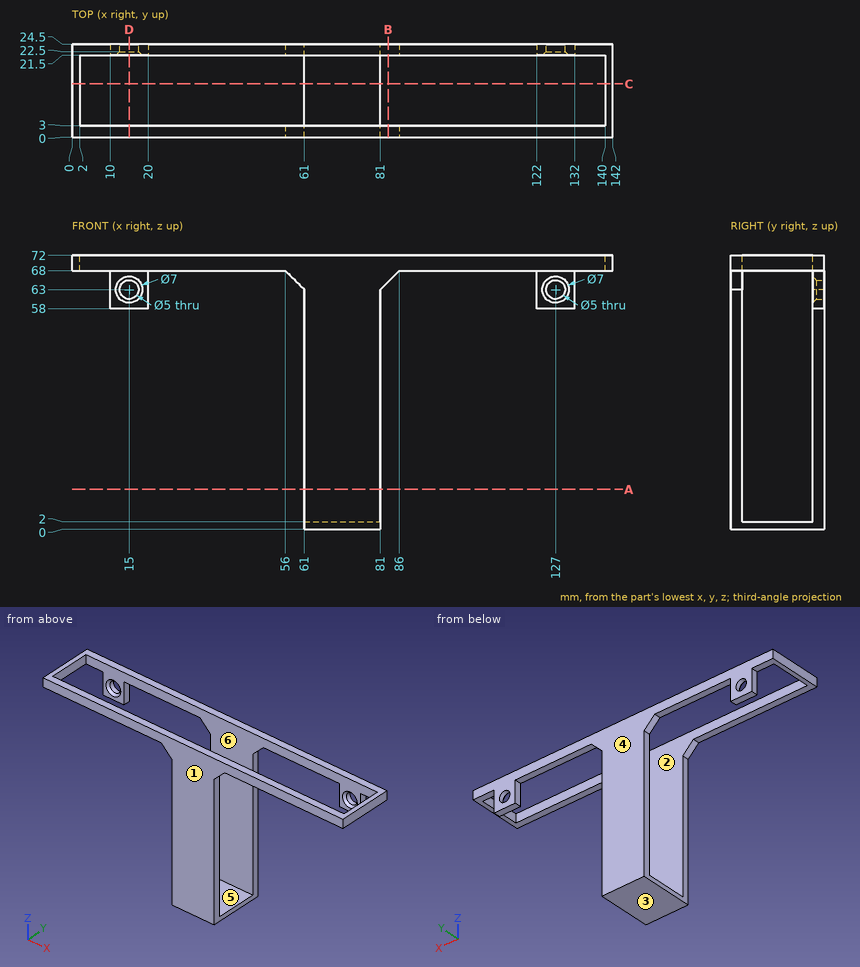
Geometry: see drawing. Coordinates: mm, zero at the bounding-box minimum. A direction names the side the tool comes from. Give positions to 0.01 mm unless a question says otherwise; leave off trailing zeros. Order: outer loops, then holes, each group sorted by start corner. A loop starts at its lowest first (then second) coordinate and runs counter-clockwise, first axis right, second up. Notation, with made-up numbers: (19.25, 84.25) -> (78.25, 84.25) arc R14 ccw to (78.25, 96.25) -> close; hole circle Ø6 at (-19, 52.5). An arc over 180 degrees is marked (long way). Write each question's results on one line, items separated by ' | '.
1) Cut plane D-D (x = 15). Output: boundary loops of the cut face in (y, z).
Geometry says:
outline: (0, 68) -> (3, 68) -> (3, 72) -> (0, 72) -> close; (21.5, 58) -> (24.5, 58) -> (24.5, 60.5) -> (22.5, 60.5) -> (21.5, 59.5) -> close; (21.5, 66.5) -> (22.5, 65.5) -> (24.5, 65.5) -> (24.5, 72) -> (21.5, 72) -> close
2) Cut plane A-A (z = 10.5). Output: boundary loops of the cut face in (x, y).
Geometry says:
outline: (61, 0) -> (81, 0) -> (81, 3) -> (61, 3) -> close; (61, 21.5) -> (81, 21.5) -> (81, 24.5) -> (61, 24.5) -> close
3) Draft query along Y for the marked faces 3, 4, 5 and 6. Return one class per face: released by +Y, released by -Y, zero draft, split by the parting line, or undercut.
Geometry says:
face 3: zero draft | face 4: released by +Y | face 5: undercut | face 6: undercut
4) First-contact query: pin 1 Ø1.5 at (x, y) = (98.5, 22.5) entering from -Z; pin 2 Ø2.5 at (y, z) = (23, 64) entering from -X; pin 3 Ø2.5 at (y, z) = (22.5, 60.5) entering from +X. Flat tips, straight axial feed; report the tip coordinate or a pass-through.
Geometry says:
pin 1: stops at z = 68 | pin 2: stops at x = 10 | pin 3: stops at x = 132
5) Line query: line 1 along X through (y, z) = (23, 63); line 2 along Z through (x, y) = (15, 23.75); line 3 along Y through (x, z) = (77.5, 27). Output: solid intervals per line, ascending.
Geometry says:
line 1: x = 10 to 12.5, 17.5 to 20, 61 to 81, 122 to 124.5, 129.5 to 132 | line 2: z = 58 to 60.5, 65.5 to 72 | line 3: y = 0 to 3, 21.5 to 24.5
6) Cut plane B-B (x = 83). Output: boundary loops of the cut face in (y, z), and give its area (3 significant figures).
Geometry says:
outline: (0, 65) -> (3, 65) -> (3, 72) -> (0, 72) -> close; (21.5, 65) -> (24.5, 65) -> (24.5, 72) -> (21.5, 72) -> close | area: 42.0 mm²
7) Set-up query: the marked faces 1 and 2. Return all of +Z, -Z, +X, -X, +Y, -Y with unobstructed straight access to the full face (end or side cutting, diameter ignored); none if empty.
Geometry says:
face 1: +Z, -Z, +X, -X, -Y | face 2: +Z
8) Cut plane C-C (y = 14). Output: boundary loops of the cut face in (x, z).
Geometry says:
outline: (0, 68) -> (2, 68) -> (2, 72) -> (0, 72) -> close; (61, 0) -> (81, 0) -> (81, 2) -> (61, 2) -> close; (140, 68) -> (142, 68) -> (142, 72) -> (140, 72) -> close
